Design review of the part built by this model. Coordinates are the model's own, in mm. Coordinates: 2 decimals unless noted, no trailing zeros. Loops run counter-clockwise (first coordinate to the right, second up) from the corner with the lowest first, then second, coordinate; pieces in that order, holes last. Notation, with made-up numbers: (-27, 23.25) - (25, 23.25) arc R19 cw to (25, 49.25) - close; hole circle Ø5 at (-2, 39.5). An arc over 180 degrees is marked (long way). One line per question, with ' | ' between items.
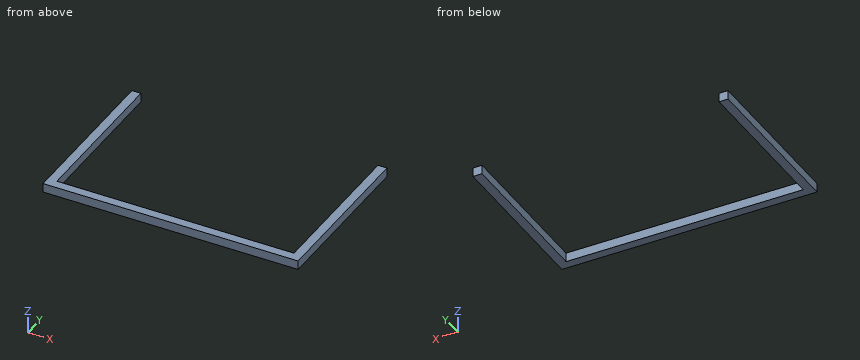
from build123d import *

# Parameters (mm, degrees)
F0_W          = 30
F0_H          = 30
F1_DEPTH      = 275
F2_W          = 30
F2_H          = 30
F3_DEPTH      = 820
F4_W          = 30
F4_H          = 30
F5_DEPTH      = 520
F5_DEPTH_BACK = 25


with BuildPart() as f1:
    # F0 (on Front) → F1 (new body, symmetric)
    with BuildSketch(Plane.XZ):
        Rectangle(F0_W, F0_H)
    extrude(amount=F1_DEPTH, both=True)

    # F2 (on face) → F3 (join)
    with BuildSketch(Plane.YZ.offset(15)):
        with Locations((-260, 0)):
            Rectangle(F2_W, F2_H)
    extrude(amount=F3_DEPTH)

    # F4 (on face) → F5 (join, two sides)
    with BuildSketch(Plane(origin=(0, -245, 0), x_dir=(-1, 0, 0), z_dir=(0, 1, 0))) as f5_sk:
        with Locations((-820, 0)):
            Rectangle(F4_W, F4_H)
    extrude(amount=F5_DEPTH)
    extrude(f5_sk.sketch, amount=-F5_DEPTH_BACK)


solid = f1.part
Q1. Take a section at B-B (z = -9.5). Give the boundary of the cut face in (x, y), plus the area to 3 significant figures.
Returned:
outline: (-15, -275) - (835, -275) - (835, 275) - (805, 275) - (805, -245) - (15, -245) - (15, 275) - (-15, 275) - close | area: 56,700 mm²
Q2. Take a section at C-C (x = 784.5). Give the boundary of the cut face in (y, z).
Returned:
outline: (-275, -15) - (-245, -15) - (-245, 15) - (-275, 15) - close
Q3. Take a section at A-A (y = 65.5). Give the boundary of the cut face in (x, z), plus the area to 3 significant figures.
Returned:
outline: (-15, -15) - (15, -15) - (15, 15) - (-15, 15) - close; (805, -15) - (835, -15) - (835, 15) - (805, 15) - close | area: 1,800 mm²
Q4. For pin 1 (4 mm diameter, centred on x = 139.5, z = -10.5, fed in from +Y), flat-tipped, find the tip position at first contact; note if it passes through.
Returned:
pin 1: stops at y = -245
Q5. To check wall thickness, follow line 1 along X through (y, z) = (-19, -7.5); line 2 along Y through (x, z) = (721, -0.5). State the ranges of each line that lie inside material, in increasing order.
Returned:
line 1: x = -15 to 15, 805 to 835 | line 2: y = -275 to -245
